Could you check a few things on this model? Use its own coordinates, in mm. A direction names the side the tool comes from. Give positions to 0.01 mm unless a question says otherwise; leave off trailing zeros. Loops run counter-clockwise (first coordinate to the right, second up) from the corner with the lowest first, then second, coordinate; pieces in that order, holes last. Notation, with made-up numbers: (74.5, -26) - (124.5, -26) arc R27 cw to (124.5, 5) - close; hole circle Ø2 at (14, 14). An arc over 180 degrees is marked (long way). Answer in a Markdown table with one row per item. Add a question column.
```python
from build123d import *

# Parameters (mm, degrees)
FILLET1_R   = 0.3048
HEX_2_DEPTH = 1.9558


with BuildPart() as part:
    # BodySke → Base-Revolve (revolve)
    with BuildSketch(Plane.XY):
        Polygon((0, 0), (0, 3.0226), (0.4064, 3.429), (4.1656, 3.429), (4.1656, 2.0828), (22.74316, 2.0828), (23.2156, 1.61036), (23.2156, 0), align=None)
    revolve(axis=Axis((-31.75, 0, 0), (1, 0, 0)))

    # Fillet1
    fillet1_edges = [part.edges().sort_by_distance(p)[0] for p in [
        (4.1656, -2.0828, 0),
    ]]
    fillet(fillet1_edges, radius=FILLET1_R)

    # Sketch3 → Hex 2 (cut)
    with BuildSketch(Plane(origin=(0, 0, 0), x_dir=(0, 0.5, 0.866025404), z_dir=(-1, 0, 0))):
        Polygon((1.026528779, 1.778), (-1.026528779, 1.778), (-2.053057557, 0), (-1.026528779, -1.778), (1.026528779, -1.778), (2.053057557, 0), align=None)
    extrude(amount=-HEX_2_DEPTH, mode=Mode.SUBTRACT)


solid = part.part
```
(1) I want a section at B-B on x = 3. Please give me the cut outline in (y, z).
(2) On a 3-axis mill with a long thin cutter (end or side, diameter ignored), from which of +Z, -Z, +X, -X, +Y, -Y can I reach the whole of each face in a straight line? I mean faces 1 (the flat face through (4.166, 1.5, -2.2)), 2 (the flat face through (1, 0, 1.778)), 3 (the flat face through (0, 0, -2)). Say none if no direction works.
(3) We'd pull the mould along Z, two halves only. Please class faces 4 (the flat face through (0.964, -1.533, -0.901)), 5 (the cylindrical face through (13.735, 1.987, 0.626)), 6 (the flat face through (23.216, 0, 0)): pulls with the +Z half, pulls with the -Z half, needs draft (parallel to the pull), parting line crosses it, or undercut.
(4) I want a section at A-A on y = 0. Please give me the cut outline in (x, z).
(5) For pin 1 Ø0.6 at (x, y) = (1, -0.5) entering from -Z; pin 2 Ø1.5 at (x, z) = (14.5, -0.5) entering from -Y; pin 3 Ø4 at (x, z) = (11.5, 0.5) entering from +Y, each with a flat end and sliding along its axis, tell me the tip position at first contact or that it passes through.
(6) Please list where these lines run through material, in increasing order: line 1 (X direction, y = 2.5, z = 0.75); line 2 (X direction, y = 0.5, z = -0.5); line 3 (Y direction, x = 7.5, z = 0.75).
Reported:
| question | item | result |
|---|---|---|
| 1 | outline | circle Ø6.86 at (0, 0) |
| 2 | face 1 | +X |
| 2 | face 2 | -X |
| 2 | face 3 | +Z, -Z, -X, +Y, -Y |
| 3 | face 4 | undercut |
| 3 | face 5 | parting line crosses it |
| 3 | face 6 | needs draft |
| 4 | outline | (0, -3.02) - (0.41, -3.43) - (4.17, -3.43) - (4.17, -2.39) arc R0.3 cw to (4.47, -2.08) - (22.74, -2.08) - (23.22, -1.61) - (23.22, 1.61) - (22.74, 2.08) - (4.47, 2.08) arc R0.3 cw to (4.17, 2.39) - (4.17, 3.43) - (0.41, 3.43) - (0, 3.02) - (0, 1.78) - (1.96, 1.78) - (1.96, -1.78) - (0, -1.78) - close |
| 5 | pin 1 | z = -3.42 |
| 5 | pin 2 | y = -2.08 |
| 5 | pin 3 | y = 2.08 |
| 6 | line 1 | 0 to 4.17 |
| 6 | line 2 | 1.96 to 23.22 |
| 6 | line 3 | -1.94 to 1.94 |
